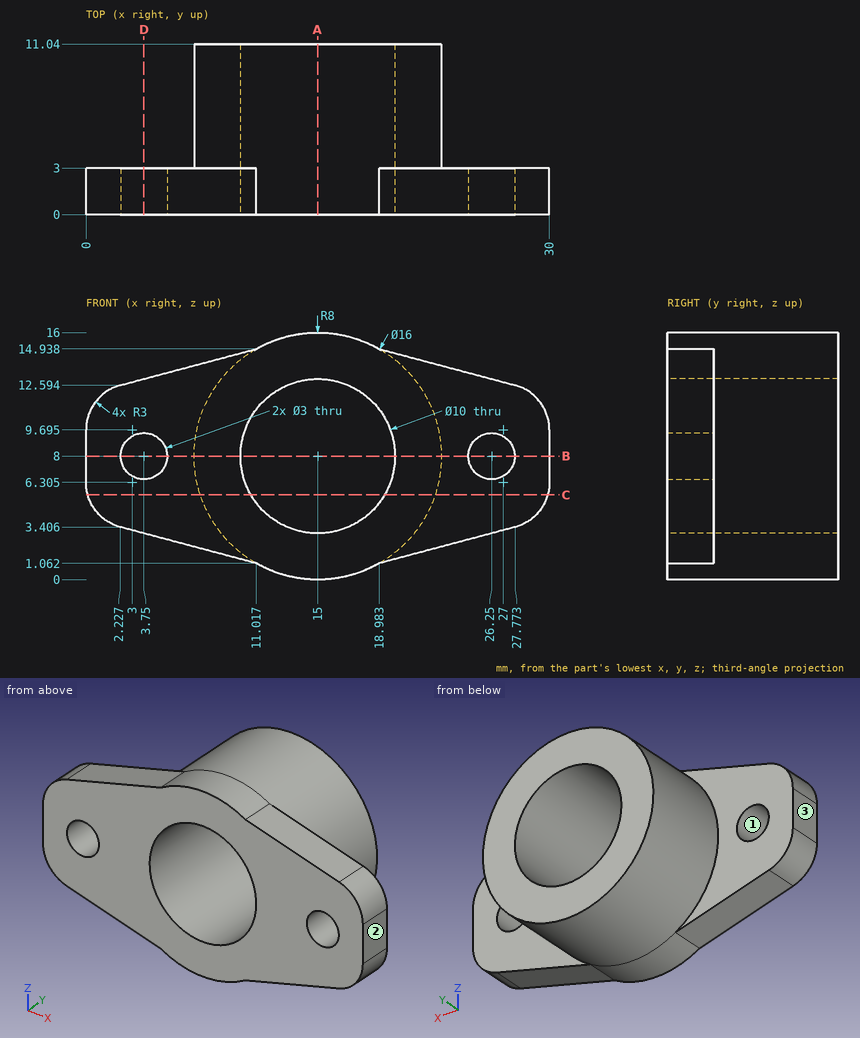
Geometry check sheet. Reference: drawing and pictorial views, mm from the part's lowest x, y, z. Coordinates: 2 decimals unless noted, no trailing zeros. Order: outer loops, then holes, each group sorted by start corner. A loop starts at its lowest first (then second) coordinate and runs counter-clockwise, first axis right, second up.
Item 1: Section check D-D, the plane x = 3.75. Enter the section's corners in (y, z), then the cut area to 3 significant figures.
Filled in:
outline: (0, 3) - (3, 3) - (3, 6.5) - (0, 6.5) - close; (0, 9.5) - (3, 9.5) - (3, 13) - (0, 13) - close
area: 21.0 mm2
Item 2: Material ranges on L1, parallel to X at y = 1.55, z = 8; L2, parallel to Z at x = 15.25, y = 1.5; L3, parallel to X at y = 10, z = 8, recorded low to high.
Filled in:
L1: x = 0 to 2.25, 5.25 to 10, 20 to 24.75, 27.75 to 30
L2: z = 0 to 3.01, 12.99 to 16
L3: x = 7 to 10, 20 to 23
Item 3: Section check A-A, the plane x = 15. Enter the section's corners in (y, z).
Filled in:
outline: (0, 0) - (11.04, 0) - (11.04, 3) - (0, 3) - close; (0, 13) - (11.04, 13) - (11.04, 16) - (0, 16) - close
Item 4: Depth check by flat-ended pin: pin 1 (8 mm diameter, centred on x = 14.5, z = 3.5, fed in from +Y); pin 2 (2 mm diameter, centred on x = 18.5, y = 2, fed in from +Z); pin 3 (2.5 mm diameter, centred on x = 26.25, z = 8, fed in from +Y); pin 4 (3 mm diameter, centred on y = 8.5, z = 4, fed in from -X). Enter the tip coordinate at first touch or a pass-through.
Filled in:
pin 1: stops at y = 11.04
pin 2: stops at z = 15.6
pin 3: passes through
pin 4: stops at x = 7.4
Item 5: Section check B-B, the plane z = 8. Enter the section's corners in (x, y).
Filled in:
outline: (0, 0) - (2.25, 0) - (2.25, 3) - (0, 3) - close; (5.25, 0) - (10, 0) - (10, 11.04) - (7, 11.04) - (7, 3) - (5.25, 3) - close; (20, 0) - (24.75, 0) - (24.75, 3) - (23, 3) - (23, 11.04) - (20, 11.04) - close; (27.75, 0) - (30, 0) - (30, 3) - (27.75, 3) - close
Item 6: Release check for a two-part mould opening along X. For the marked faces 1, 2 and 3 record: +X half, -X half, draft (parallel to the pull), parting line (faces both ways), or undercut.
Filled in:
face 1: undercut
face 2: +X half
face 3: -X half
Item 7: Section check C-C, the plane z = 5.5. Enter the section's corners in (x, y), then the cut area to 3 significant figures.
Filled in:
outline: (0.11, 0) - (10.67, 0) - (10.67, 11.04) - (7.4, 11.04) - (7.4, 3) - (0.11, 3) - close; (19.33, 0) - (29.89, 0) - (29.89, 3) - (22.6, 3) - (22.6, 11.04) - (19.33, 11.04) - close
area: 116 mm2
